Autodesk Inventor part; units mm, degrees
ref_plane "YZ Plane" through (0, 0, 0) normal (1, 0, 0) x (0, 1, 0)
ref_plane "XZ Plane" through (0, 0, 0) normal (0, 1, 0) x (-1, 0, 0)
ref_plane "XY Plane" through (0, 0, 0) normal (0, 0, 1) x (1, 0, 0)
sketch "Sketch1" plane through (0, 0, 0) normal (1, 0, 0) x (0, 1, 0)
  circle A0 centre (0, 0) radius 3.683
  line L0 (4.699, 2.6924) -> (0, 2.6924)
  line L1 (0, 2.6924) -> (0, -2.6924)
  line L2 (0, -2.6924) -> (4.699, -2.6924)
  line L3 (4.699, -2.6924) -> (4.699, 2.6924)
  dimension "d0" = 7.366
  dimension "d1" = 5.3848
  dimension "d2" = 4.699
extrude "Extrusion1" add sketch "Sketch1" along normal blind 0.635
fillet "Fillet1" radius 5.08 2 edges at (0.3175, 2.5131, -2.6924) (0.3175, 2.5131, 2.6924)
sketch "Sketch2" plane through (0.635, 0, 0) normal (1, 0, 0) x (0, 0, -1)
  arc A0 (-3.2667, 1.701) -> (3.2667, 1.701) centre (0, 0) ccw
  line L0 (2.6924, 4.699) -> (-2.6924, 4.699)
  circle A1 centre (0, 0) radius 2.921
  line L1 (-0.635, 2.8511) -> (0.635, 2.8511)
  line L2 (0.635, 2.8511) -> (0.635, 4.699)
  line L3 (0.635, 4.699) -> (-0.635, 4.699)
  line L4 (-0.635, 4.699) -> (-0.635, 2.8511)
  dimension "d6" = 5.842
  dimension "d7" = 1.27
extrude "Extrusion2" cut sketch "Sketch2" against normal through all
sketch "Sketch3" plane through (0.635, 0, 0) normal (1, 0, 0) x (0, 0, -1)
  line L0 (-0.635, 2.8511) -> (-2.6924, 4.699) construction
  line L1 (0.635, 2.8511) -> (2.6924, 4.699) construction
  point P0 (-1.6637, 3.7751)
  point P1 (1.6637, 3.7751)
hole "Hole1" at (0.635, 3.7751, 1.6637) at (0.635, 3.7751, -1.6637) direction (-1, 0, 0) diameter 1.27 end through all
properties part number "Horseshoe Clip"
The model under review builds one solid part; all positions refer to its coordinate system, in mm. Give positions to 0.01 mm unless a question says otherwise; leave off trailing zeros. Write each loop counter-clockwise with the first axis right and the second up, starting at its lowest first coordinate (ties: lowest second). Pieces come first, ordered by that corner, then holes. Notation, with made-up numbers: (70.25, 28) - (88.25, 28) arc R26 cw to (88.25, 66) - close; hole circle Ø4 at (-30.75, -13.75). An arc over 180 degrees is marked (long way). Answer in a Markdown table with one row per item. Add a question column.
1. We need section C-C on x = 0.4. Write out the cut boundary in (y, z) (3 decimals).
2. We need section D-D on y = 3.5. Write out the cut boundary in (x, z) (3 decimals), then the cut area to 3 significant figures.
3. Draft analysis for pull direction Y (two halves, no side actions). For faces 1 (the cylindrical face through (0.313, 4.395, 1.801)), 2 (the cylindrical face through (0.31, -3.68, -0.11)), 3 (the flat face through (0, 3, 1)), state which applies: +Y half, -Y half, draft (parallel to the pull), parting line (faces both ways), or undercut.
4. Insertion check: P1, Ø0.8, axis at y = 3.78, z = -1.66, coming from the -X side; P2, Ø2, axis at y = 3.78, z = 1.66, coming from the +X side (3 decimals). Each pin has a flat end and moves straight along its axis. Give the tip position at first contact, or say it passes through.
5. Wall thickness on line 1 along Y through (x, z) = (0.2, -2); line 2 along Z through (x, y) = (0.45, 0); line 3 along Z through (x, y) = (0.4, 4) (3 decimals): over which ranges is each line inside the solid? List them lowest first. Write a range as [from, to].
6. We need section A-A on y = 0. Write out the cut boundary in (x, z) (3 decimals), then the cut area to 3 significant figures.
7. We need section B-B on z = 1.25. Write out the cut boundary in (x, y) (3 decimals), then the cut area to 3 significant figures.
Ans:
| question | item | result |
|---|---|---|
| 1 | outline | (1.701, -3.267) arc R5.08 cw to (4.047, -2.692) - (4.699, -2.692) - (4.699, -0.635) - (2.851, -0.635) arc R2.921 cw (long way) to (2.851, 0.635) - (4.699, 0.635) - (4.699, 2.692) - (4.047, 2.692) arc R5.08 cw to (1.701, 3.267) arc R3.683 ccw (long way) to start; hole circle Ø1.27 at (3.775, -1.664); hole circle Ø1.27 at (3.775, 1.664) |
| 2 | outline | (0, -2.722) - (0.635, -2.722) - (0.635, -2.236) - (0, -2.236) - close; (0, -1.091) - (0.635, -1.091) - (0.635, -0.635) - (0, -0.635) - close; (0, 0.635) - (0.635, 0.635) - (0.635, 1.091) - (0, 1.091) - close; (0, 2.236) - (0.635, 2.236) - (0.635, 2.722) - (0, 2.722) - close |
| 2 | area | 1.20 mm^2 |
| 3 | face 1 | undercut |
| 3 | face 2 | parting line |
| 3 | face 3 | draft |
| 4 | P1 | passes through |
| 4 | P2 | stops at x = 0.635 |
| 5 | line 1 | y = [-3.09, -2.13], [2.13, 3.24], [4.31, 4.7] |
| 5 | line 2 | z = [-3.68, -2.92], [2.92, 3.68] |
| 5 | line 3 | z = [-2.693, -2.258], [-1.07, -0.635], [0.635, 1.07], [2.258, 2.693] |
| 6 | outline | (0, -3.683) - (0.635, -3.683) - (0.635, -2.921) - (0, -2.921) - close; (0, 2.921) - (0.635, 2.921) - (0.635, 3.683) - (0, 3.683) - close |
| 6 | area | 0.968 mm^2 |
| 7 | outline | (0, -3.464) - (0.635, -3.464) - (0.635, -2.64) - (0, -2.64) - close; (0, 2.64) - (0.635, 2.64) - (0.635, 3.293) - (0, 3.293) - close; (0, 4.257) - (0.635, 4.257) - (0.635, 4.699) - (0, 4.699) - close |
| 7 | area | 1.22 mm^2 |
